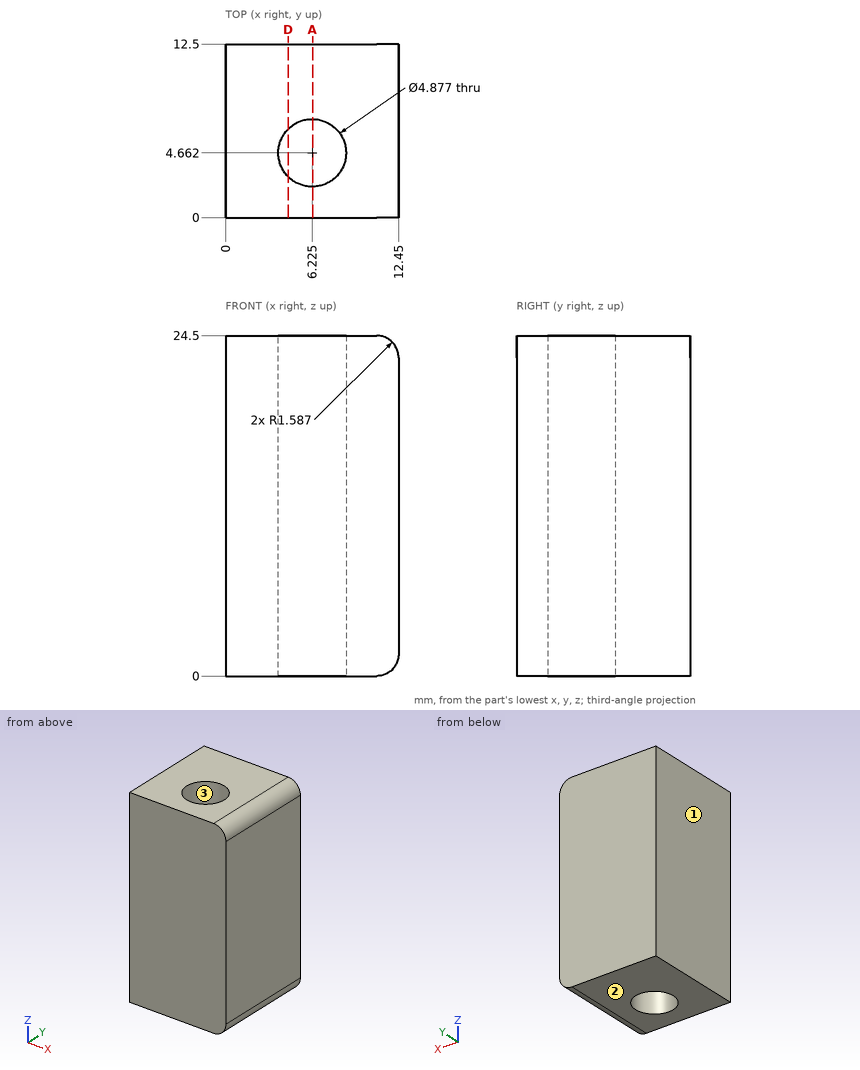
Design review of the part shown in the three views and the two pictorial views. Dimensions are in mm from the part's minimum x, y and z. Round coordinates to 2 decimals unless told otherwise and drop trailing zeros. Write each loop counter-clockwise with the first axis right and the second up, starting at its lowest first coordinate (ties: lowest second). Pieces come first, ordered by that corner, then holes. Notation, with made-up numbers: (31.25, -20.5) -> (63.25, -20.5) arc R12 cw to (63.25, -12.5) -> close; hole circle Ø9 at (27, 61.5). An arc over 180 degrees is marked (long way). Answer as a JSON object with one key per item and string values.
1. The part is to be moulded in two halves that separate along X. For the marked faces 1, 2 and 3, say which applies: pulls with the +X half, pulls with the -X half, needs draft (parallel to the pull), parting line crosses it, or undercut.
Results found:
{"face 1": "pulls with the -X half", "face 2": "needs draft", "face 3": "undercut"}
2. To check wall thickness, follow line 1 along X through (y, z) = (5, 8.25); line 2 along Y through (x, z) = (7.5, 11.25) (1 decimal); line 3 along Y through (x, z) = (6.5, 18.25) (1 decimal). State the ranges of each line that lie inside material, in increasing order.
Results found:
{"line 1": "x = 0 to 3.81, 8.64 to 12.45", "line 2": "y = 0 to 2.6, 6.7 to 12.5", "line 3": "y = 0 to 2.2, 7.1 to 12.5"}
3. We need section D-D on x = 4.5. State the section outline as (y, z) points (1 decimal), and give its area (3 significant figures).
Results found:
{"outline": "(0, 0) -> (2.9, 0) -> (2.9, 24.5) -> (0, 24.5) -> close; (6.4, 0) -> (12.5, 0) -> (12.5, 24.5) -> (6.4, 24.5) -> close", "area": "222 mm^2"}
4. We need section A-A on x = 6.25. State the section outline as (y, z) points (1 decimal).
Results found:
{"outline": "(0, 0) -> (2.2, 0) -> (2.2, 24.5) -> (0, 24.5) -> close; (7.1, 0) -> (12.5, 0) -> (12.5, 24.5) -> (7.1, 24.5) -> close"}
